Source: three-view drawing plus pictorial views. Frame: mm from the lowest corner of the part. Coordinates: 2 decimals unless noted, no trailing zeros. Write each loop counter-clockwise with the first axis right and the second up, starting at its lowest first coordinate (ties: lowest second). Pieces come first, ordered by that corner, then holes. Notation, with made-up numbers: (31, 40.25) - (65, 40.25) arc R26 ccw to (65, 72.25) - close; hole circle Ø3 at (65, 17.5). An arc over 180 degrees is marked (long way). One line per item, written item: value.
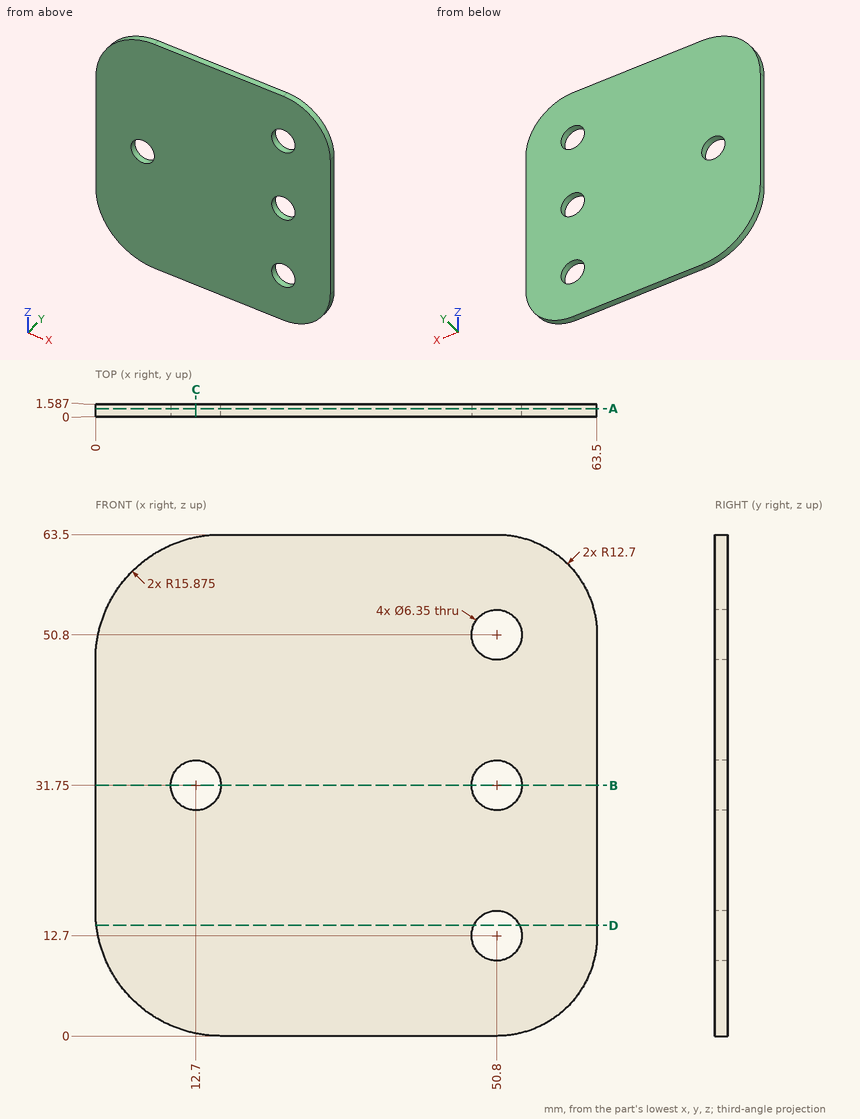
1) Section query C-C on x = 12.7. Output: boundary loops of the cut face in (y, z) (1 decimal).
Values found:
outline: (0, 0.3) - (1.6, 0.3) - (1.6, 28.6) - (0, 28.6) - close; (0, 34.9) - (1.6, 34.9) - (1.6, 63.2) - (0, 63.2) - close
2) Material intervals for line 1 (X direction, y = 0.4, z = 31.75) (1 decimal); line 2 (Z direction, x = 50.8, y = 1.2) (1 decimal); line 3 (Z direction, x = 12.7, y = 0.55) (1 decimal), sorted ascending.
Values found:
line 1: 0 to 9.5, 15.9 to 47.6, 54 to 63.5
line 2: 0 to 9.5, 15.9 to 28.6, 34.9 to 47.6, 54 to 63.5
line 3: 0.3 to 28.6, 34.9 to 63.2
3) Section query D-D on z = 14. Output: boundary loops of the cut face in (x, y).
Values found:
outline: (0.11, 0) - (47.9, 0) - (47.9, 1.59) - (0.11, 1.59) - close; (53.7, 0) - (63.5, 0) - (63.5, 1.59) - (53.7, 1.59) - close
4) Section query A-A on y = 1. State how many separate pieces and enclosed holes the cut face has, then the cut area to 3 significant figures.
Values found:
separate pieces: 1
enclosed holes: 4
area: 3,730 mm2
5) Section query B-B on z = 31.75. Output: boundary loops of the cut face in (x, y) (1 decimal).
Values found:
outline: (0, 0) - (9.5, 0) - (9.5, 1.6) - (0, 1.6) - close; (15.9, 0) - (47.6, 0) - (47.6, 1.6) - (15.9, 1.6) - close; (54, 0) - (63.5, 0) - (63.5, 1.6) - (54, 1.6) - close
6) Contact query for a flat-ended pin moving along its axis: P1, Ø5.5, axis at x = 50.8, z = 31.75, coming from the -Y side. Output: stop coordinate, or through.
Values found:
P1: through
